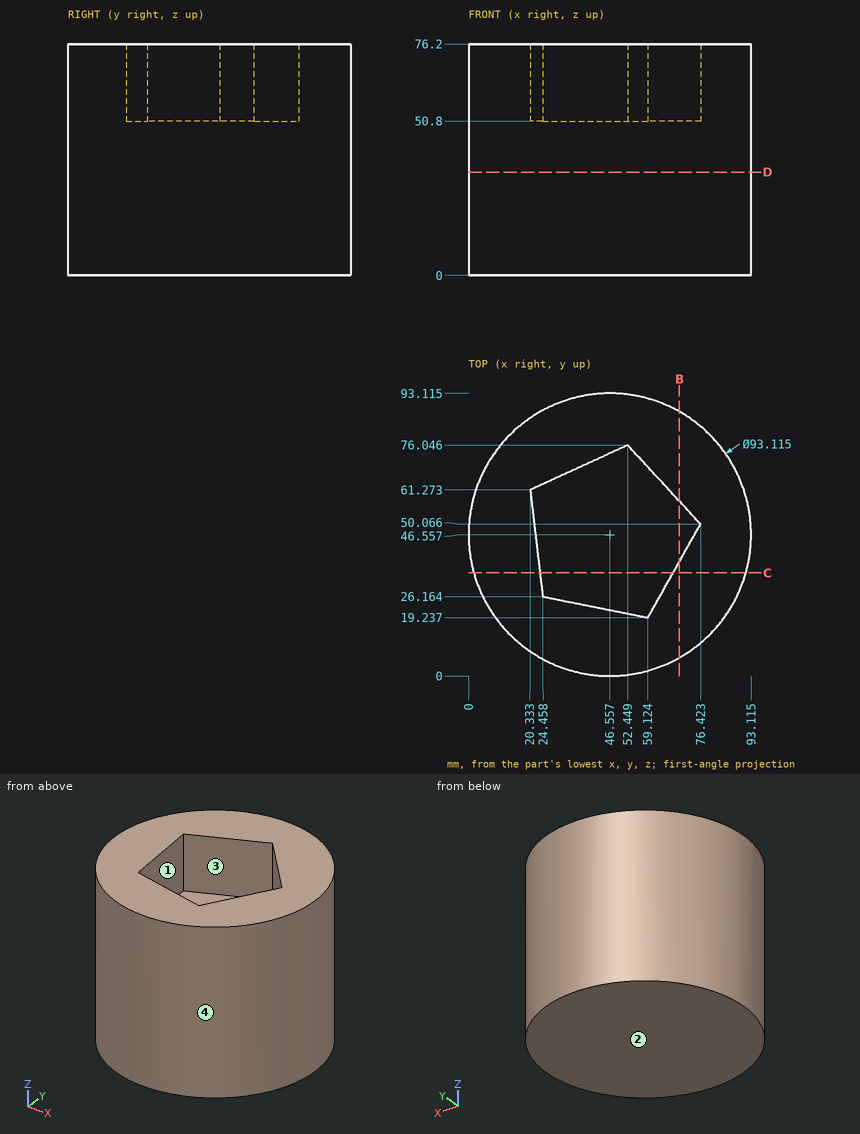
Source: three-view drawing plus pictorial views. Frame: mm from the lowest corner of the part. Round coordinates to 2 decimals unless told otherwise and drop trailing zeros. Order: outer loops, then holes, each group sorted by start corner. A loop starts at its lowest first (then second) coordinate and runs counter-clockwise, first axis right, second up. Notation, with made-up numbers: (31, -33) - (68, -33) arc R13 ccw to (68, -8) - close; hole circle Ø9 at (28.25, 82). An arc over 180 degrees is marked (long way). Write each question's results on one line, items separated by ' | '.
Item 1: Mould query, pull axis Y, two halves, no side actions, for the marked faces 1, 2, 3 and 4. Classes: pulls with the +Y half, pulls with the -Y half, needs draft (parallel to the pull), parting line crosses it, or undercut.
Completed:
face 1: undercut | face 2: needs draft | face 3: undercut | face 4: parting line crosses it
Item 2: Section D-D, the plane z = 34. Return the cut outline in (x, y) (1 decimal), and give its area (3 significant figures).
Completed:
outline: circle Ø93.1 at (46.6, 46.6) | area: 6,810 mm^2
Item 3: Section C-C, the plane y = 34. Return the cut outline in (x, z) (1 decimal), and give its area (3 significant figures).
Completed:
outline: (1.7, 0) - (91.4, 0) - (91.4, 76.2) - (67.4, 76.2) - (67.4, 50.8) - (23.5, 50.8) - (23.5, 76.2) - (1.7, 76.2) - close | area: 5,720 mm^2
Item 4: Material intervals for line 1 along Z through (x, y) = (54, 22.5); line 2 along Y through (x, z) = (45, 33); line 3 along Y through (x, z) = (37, 61), sorted ascending. Write a range as [from, to].
Completed:
line 1: [0, 50.8] | line 2: [0.03, 93.09] | line 3: [0.99, 23.66], [68.94, 92.12]
Item 5: Section B-B, the plane x = 69.5. Return the cut outline in (y, z) (1 decimal).
Completed:
outline: (6, 0) - (87.1, 0) - (87.1, 76.2) - (57.6, 76.2) - (57.6, 50.8) - (37.7, 50.8) - (37.7, 76.2) - (6, 76.2) - close
Item 6: First-contact query: pin 1 Ø6 at (y, z) = (75, 45.5) entering from -X; pin 2 Ø1.5 at (y, z) = (24.5, 24.5) entering from +X; pin 3 Ø5 at (x, z) = (25, 62.5) entering from -Y. Flat tips, straight axial feed; report the tip coordinate or a pass-through.
Completed:
pin 1: x = 7.57 | pin 2: x = 87.95 | pin 3: y = 4.08
